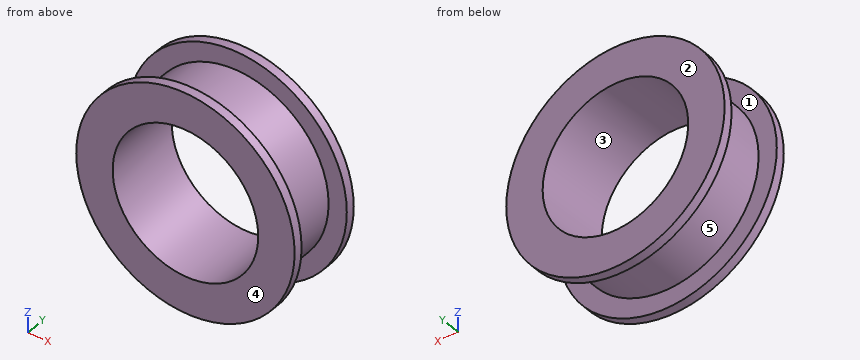
Autodesk Fusion 360 part; units mm, degrees
sketch "Sketch1" plane through (0, 0, 0) normal (0, 0, 1) x (1, 0, 0)
  line L0 (0, 0) -> (8, 0) construction
  line L1 (8, 0) -> (8, 8.5)
  line L2 (8, 8.5) -> (12, 8.5)
  line L3 (12, 8.5) -> (12, 7.5)
  line L4 (12, 7.5) -> (10, 7.5)
  line L5 (10, 7.5) -> (10, 1)
  line L6 (10, 1) -> (12, 1)
  line L7 (12, 1) -> (12, 0)
  line L8 (12, 0) -> (8, 0)
  dimension "d1" = 1
  dimension "d2" = 1
  dimension "d3" = 6.5
  dimension "d4" = 8
  dimension "d5" = 2
  dimension "d6" = 2
revolve "Revolve1" add sketch "Sketch1" angle 360 about axis through (0, 1.75, 0) along (0, 1, 0)
The listing builds one solid part. Answer for the finished solid, in the listing's coordinates (mm). Face numbers are marked on the shaded views. A direction names the side the tool comes from. Give positions to 0.01 mm unless a question says otherwise; leave off trailing zeros. Loops run counter-clockwise (first coordinate to the right, second up) from the corner with the lowest first, then second, coordinate; pieces in that order, holes last. Notation, with made-up numbers: (18.25, -16) - (34.25, -16) arc R23 cw to (34.25, 20) - close; hole circle Ø7 at (3, 37.5). An arc over 180 degrees is marked (long way). Answer as a JSON object with one key per item and string values.
1. A cutting plane is placed at A-A (x = 0). Write down the section's boundary in (y, z), then the cut area to 3 significant figures.
Determined:
{"outline": "(0, -12) - (1, -12) - (1, -10) - (7.5, -10) - (7.5, -12) - (8.5, -12) - (8.5, -8) - (0, -8) - close; (0, 8) - (8.5, 8) - (8.5, 12) - (7.5, 12) - (7.5, 10) - (1, 10) - (1, 12) - (0, 12) - close", "area": "42.0 mm²"}
2. A cutting plane is placed at C-C (y = 6). Write down the section's boundary in (x, z).
Determined:
{"outline": "circle Ø20 at (0, 0); hole circle Ø16 at (0, 0)"}
3. A cutting plane is placed at B-B (z = 0). Write down the section's boundary in (x, y), then the cut area to 3 significant figures.
Determined:
{"outline": "(-12, 0) - (-8, 0) - (-8, 8.5) - (-12, 8.5) - (-12, 7.5) - (-10, 7.5) - (-10, 1) - (-12, 1) - close; (8, 0) - (12, 0) - (12, 1) - (10, 1) - (10, 7.5) - (12, 7.5) - (12, 8.5) - (8, 8.5) - close", "area": "42.0 mm²"}
4. Find the intervals of material crossed by L1, parallel to X at y = 2, z = 0; L2, parallel to Y at x = 4.25, z = 10.5, in increasing order. Write a range as [from, to].
Determined:
{"L1": "[-10, -8], [8, 10]", "L2": "[0, 1], [7.5, 8.5]"}
5. For a pull along Y with two mould halves and no side action, classify the marked faces 3, 4 and 5 as pulls with the +Y half, pulls with the -Y half, needs draft (parallel to the pull), parting line crosses it, or undercut.
Determined:
{"face 3": "needs draft", "face 4": "pulls with the -Y half", "face 5": "undercut"}
6. For the marked faces 1 and 2, determine the directions among +Z, -Z, +X, -X, +Y, -Y from which every point of the face is accessible in a straight line to the end or side of a thin tool.
Determined:
{"face 1": "none", "face 2": "+Z, -Z, +X, -X, +Y"}
7. Flat-ended cylindrical pins translate along their axes: pin 1 Ø3 at (y, z) = (6.5, 6.5) entering from +X; pin 2 Ø3 at (y, z) = (6.5, 4.5) entering from +X; pin 3 Ø3 at (x, y) = (-1.5, 4.5) entering from +Z; pin 4 Ø2 at (x, z) = (-4, -4) entering from +Y. Find the tip coordinate at first contact, or state that the pin passes through.
Determined:
{"pin 1": "x = 10.73", "pin 2": "x = 11.51", "pin 3": "z = 10", "pin 4": "through"}
